Design review of the part built by this model. Coordinates are the model's own, in mm. A direction names the side the tool comes from. Coordinates: 2 decimals unless noted, no trailing zeros. Write each loop counter-clockwise with the first axis right and the second up, starting at its lowest first coordinate (ties: lowest second). Pieces come first, ordered by that corner, then holes. Notation, with made-up numbers: (39, 89.5) - (87, 89.5) arc R18 cw to (87, 121.5) - close; hole circle Ø2 at (59, 86). An arc over 180 degrees is marked (long way). Answer as a JSON object with one key per item and string values.
```python
from build123d import *

# Parameters (mm, degrees)
FILLET2_R     = 0.1
SKETCH2_W     = 5.5
SKETCH2_H     = 0.8
SLOT_DEPTH    = 0.85
CHAMFER1_SIZE = 0.2


with BuildPart() as part:
    # BodySke → Base-Revolve (revolve)
    with BuildSketch(Plane.XY, mode=Mode.PRIVATE) as base_revolve_sk:
        Polygon((2, 1.5), (2, 2.75), (0, 2.575022673), (0, 0), (39, 0), (39, 1.5), align=None)
    revolve(base_revolve_sk.sketch.rotate(Axis((-25.4, 0, 0), (1, 0, 0)), 90), axis=Axis((-25.4, 0, 0), (1, 0, 0)))

    # Fillet2
    fillet2_edges = [part.edges().sort_by_distance(p)[0] for p in [
        (0, 0, -2.575022673),
    ]]
    fillet(fillet2_edges, radius=FILLET2_R)

    # Sketch2 → Slot (cut)
    with BuildSketch(Plane(origin=(0, 0, 0), x_dir=(0, 0, -1), z_dir=(1, 0, 0))):
        Rectangle(SKETCH2_W, SKETCH2_H)
    extrude(amount=SLOT_DEPTH, mode=Mode.SUBTRACT)

    # Chamfer1
    chamfer1_edges = [part.edges().sort_by_distance(p)[0] for p in [
        (39, 0, -1.5),
    ]]
    chamfer(chamfer1_edges, length=CHAMFER1_SIZE)


solid = part.part
```
(1) Take a section at C-C, the plane x = 10.5. Write out the cut boundary in (y, z).
Solved:
{"outline": "circle Ø3 at (0, 0)"}
(2) To check wall thickness, follow line 1 (X direction, y = 2.4, z = -0.5); line 2 (X direction, y = 0.15, z = -0.7); line 3 (Z direction, x = 10, y = -0.15). State the ranges of each line that lie inside material, in increasing order. Write a range as from..to.
Solved:
{"line 1": "x = 0..2", "line 2": "x = 0.85..39", "line 3": "z = -1.49..1.49"}
(3) Take a section at A-A, the plane y = 0. Write out the cut boundary in (x, z), and give its area (3 significant figures).
Solved:
{"outline": "(0.85, -2.65) - (2, -2.75) - (2, -1.5) - (38.8, -1.5) - (39, -1.3) - (39, 1.3) - (38.8, 1.5) - (2, 1.5) - (2, 2.75) - (0.85, 2.65) - close", "area": "117 mm^2"}
(4) Take a section at B-B, the plane z = 0. Write out the cut boundary in (x, y), and give its area (3 significant figures).
Solved:
{"outline": "(0, -2.48) arc R0.1 ccw to (0.09, -2.58) - (2, -2.75) - (2, -1.5) - (38.8, -1.5) - (39, -1.3) - (39, 1.3) - (38.8, 1.5) - (2, 1.5) - (2, 2.75) - (0.09, 2.58) arc R0.1 ccw to (0, 2.48) - (0, 0.4) - (0.85, 0.4) - (0.85, -0.4) - (0, -0.4) - close", "area": "121 mm^2"}
(5) The part is to be moulded in two halves that separate along Y. For faces 4 (the face through (0, -1, 0)), 5 (the face through (0.4, -0.4, 0)), 6 (the face through (0.82, 1.014, 2.445)), say which applies: pulls with the +Y half, pulls with the -Y half, needs draft (parallel to the pull), parting line crosses it, or undercut.
Solved:
{"face 4": "needs draft", "face 5": "undercut", "face 6": "parting line crosses it"}
(6) Tool access review of faces 1 (the face through (2, 1.2, -1.2)), 2 (the face through (0.85, 0, 0)), 3 (the face through (0, 1, 0)): name each direction out of +Z, -Z, +X, -X, +Y, -Y from which nothing blocks a thin tool from reaching the whole face with its end or side.
Solved:
{"face 1": "+X", "face 2": "+Z, -Z, -X", "face 3": "+Z, -Z, -X, +Y, -Y"}
(7) For pin 1 (3 mm diameter, centred on x = 16.5, y = -0.5, fed in from +Z); pin 2 (2 mm diameter, centred on x = 12, z = -1.5, fed in from +Y); pin 3 (0.7 mm diameter, centred on x = 0.5, z = 1.5, fed in from -Y), all flat-tipped, find the tip position at first contact; note any pin that passes through.
Solved:
{"pin 1": "stops at z = 1.5", "pin 2": "stops at y = 1.41", "pin 3": "stops at y = -2.36"}
